Build history of the part. All positions in model axes, mm. Round coordinates to 2 decimals unless told otherwise and drop trailing zeros. Write each loop counter-clockwise with the first axis right and the second up, starting at its lowest first coordinate (ties: lowest second). Pieces come first, ordered by that corner, then holes. Notation, with made-up numbers: M 10.5,71.25 L 63.5,71.25 A15 ccw 63.5,88.25 Z; hole C 23.5,-34.75 d5. An arc over 180 degrees is marked long. Write item = value, one per line.
from build123d import *

# Parameters (mm, degrees)
CHAMFER1_SIZE = 0.254


with BuildPart() as part:
    # Sketch1 → Revolve1 (revolve)
    with BuildSketch(Plane.XY):
        with BuildLine():
            Line((0, 2.7686), (12.7, 2.7686))
            Line((12.7, 2.7686), (12.7, 2.0066))
            Line((12.7, 2.0066), (4.3434, 2.0066))
            ThreePointArc((4.3434, 2.0066), (4.81222687, 1.251446675), (4.992165092, 0.381))
            Line((4.992165092, 0.381), (4.484165092, 0.381))
            ThreePointArc((4.484165092, 0.381), (4.30422687, 1.251446675), (3.8354, 2.0066))
            Line((3.8354, 2.0066), (0, 2.0066))
            Line((0, 2.0066), (0, 2.7686))
        make_face()
    revolve(axis=Axis((-4.561757333, 0, 0), (1, 0, 0)))

    # Chamfer1
    chamfer1_edges = [part.edges().sort_by_distance(p)[0] for p in [
        (12.7, -2.0066, 0),
    ]]
    chamfer(chamfer1_edges, length=CHAMFER1_SIZE)


solid = part.part
1. Band-saw the part on B-B (y = 2.4). List the corners of the cut face in (x, z).
Responses:
outline = M 0,-1.38 L 12.7,-1.38 L 12.7,1.38 L 0,1.38 Z
2. Flat gauge pins, fed straight in: pin 1 (3 mm diameter, centred on x = 8, y = -0.5, fed in from +Z); pin 2 (1.5 mm diameter, centred on x = 1.5, z = 1.5, fed in from -Y); pin 3 (1.5 mm diameter, centred on x = 6, y = 1.5, fed in from -Z). Where does each tip first touch, or does it go through?
Responses:
pin_1 = 2.77
pin_2 = -2.67
pin_3 = -2.67
3. Probe probe 1 along Z at (x, y) = (2, 0); probe 2 along Z at (x, y) = (9.75, -1.35); probe 3 along Y at (x, z) = (7.5, 1.45). List the from-to ranges inside material, lowest first.
Responses:
probe_1 = -2.77 to -2.01, 2.01 to 2.77
probe_2 = -2.42 to -1.48, 1.48 to 2.42
probe_3 = -2.36 to -1.39, 1.39 to 2.36
4. Mould opens along Y. For faces 1 (the face through (0, -2, 1)), 2 (the face through (6.44, -2.2, -1.68)), 3 (the face through (8.338, -1.479, 1.356)) say: pulls with the +Y half, pulls with the -Y half, needs draft (parallel to the pull), parting line crosses it, or undercut.
Responses:
face_1 = needs draft
face_2 = parting line crosses it
face_3 = undercut
5. Band-saw the part on A-A (x = 11.5). List the corners of the cut face in (y, z).
Responses:
outline = C 0,0 d5.54; hole C 0,0 d4.01
